from build123d import *

# Parameters (mm, degrees)
SKETCH1_R           = 1.6
BOSS_EXTRUDE1_DEPTH = 3
SKETCH2_W           = 10
SKETCH2_H           = 10
BOSS_EXTRUDE2_DEPTH = 42
CHAMFER1_SIZE       = 5
SKETCH3_R           = 2.1
CUT_EXTRUDE1_DEPTH  = 52
SKETCH4_R           = 2.65
CUT_EXTRUDE2_DEPTH  = 0.5
SKETCH5_W           = 3
SKETCH5_H           = 43
BOSS_EXTRUDE3_DEPTH = 75
SKETCH6_W           = 3
SKETCH6_H           = 72.7
BOSS_EXTRUDE4_DEPTH = 2
SKETCH7_W           = 3
SKETCH7_H           = 68.8
BOSS_EXTRUDE5_DEPTH = 3
BOSS_EXTRUDE7_DEPTH = 8.2
SKETCH9_W           = 12
SKETCH9_H           = 19.5
CUT_EXTRUDE3_DEPTH  = 8.5
SKETCH10_W          = 3
SKETCH10_H          = 56.8
BOSS_EXTRUDE8_DEPTH = 15
SKETCH13_W          = 3
SKETCH13_H          = 56.8
BOSS_EXTRUDE9_DEPTH = 45
SKETCH14_R          = 1.5
SKETCH14_R_2        = 5.5
CUT_EXTRUDE4_DEPTH  = 10
CAVITY2_START       = 23.487603306
CAVITY2_OUTLINE_R   = 2
CAVITY2_DEPTH       = 2


# Read off the part's stored shape, not the designer's step: Cavity2
with BuildPart() as part:
    # Sketch1 → Boss-Extrude1 (new body)
    with BuildSketch(Plane(origin=(0, 0, 0), x_dir=(1, 0, 0), z_dir=(0, 1, 0))):
        Polygon((-6.512396694, 9.685950413), (1.487603306, 9.685950413), (26.487603306, 9.685950413), (26.487603306, -40.314049587), (1.487603306, -40.314049587), (-6.512396694, -40.314049587), align=None)
        with Locations(Location((-1.962396694, -35.764049587, 0), (0, 0, 270))):
            Circle(SKETCH1_R, mode=Mode.SUBTRACT)
        with Locations(Location((-1.962396694, 5.135950413, 0), (0, 0, 270))):
            Circle(SKETCH1_R, mode=Mode.SUBTRACT)
    extrude(amount=BOSS_EXTRUDE1_DEPTH)

    # Sketch2 → Boss-Extrude2 (add)
    with BuildSketch(Plane(origin=(0, 3, 0), x_dir=(1, 0, 0), z_dir=(0, 1, 0))):
        with Locations((21.487603306, -35.314049587)):
            Rectangle(SKETCH2_W, SKETCH2_H)
        with Locations((21.487603306, 4.685950413)):
            Rectangle(SKETCH2_W, SKETCH2_H)
    extrude(amount=BOSS_EXTRUDE2_DEPTH)

    # Chamfer1
    chamfer1_edges = [part.edges().sort_by_distance(p)[0] for p in [
        (21.487603306, 3, 30.314049587),
        (16.487603306, 3, 35.314049587),
        (16.487603306, 3, -4.685950413),
        (21.487603306, 3, 0.314049587),
    ]]
    chamfer(chamfer1_edges, length=CHAMFER1_SIZE)

    # Sketch3 → Cut-Extrude1 (cut)
    with BuildSketch(Plane(origin=(0, 45, 0), x_dir=(1, 0, 0), z_dir=(0, 1, 0))):
        with Locations(Location((22.537603306, -36.364049587, 0), (0, 0, 270))):
            Circle(SKETCH3_R)
        with Locations(Location((22.537603306, 5.735950413, 0), (0, 0, 270))):
            Circle(SKETCH3_R)
    extrude(amount=-CUT_EXTRUDE1_DEPTH, mode=Mode.SUBTRACT)

    # Sketch4 → Cut-Extrude2 (cut)
    with BuildSketch(Plane(origin=(0, 45, 0), x_dir=(1, 0, 0), z_dir=(0, 1, 0))):
        with Locations(Location((22.537603306, -36.364049587, 0), (0, 0, 270))):
            Circle(SKETCH4_R)
        with Locations(Location((22.537603306, 5.735950413, 0), (0, 0, 270))):
            Circle(SKETCH4_R)
    cut_extrude2 = extrude(amount=-CUT_EXTRUDE2_DEPTH, mode=Mode.SUBTRACT)

    # Mirror1: Cut-Extrude2 across plane
    add(cut_extrude2.mirror(Plane(origin=(0, 22.5, 0), x_dir=(0, 0, 1), z_dir=(0, -1, 0))), mode=Mode.SUBTRACT)

    # Sketch5 → Boss-Extrude3 (add)
    with BuildSketch(Plane(origin=(0, 0, -9.685950413), x_dir=(-1, 0, 0), z_dir=(0, 0, -1))):
        with Locations((-24.987603306, 21.5)):
            Rectangle(SKETCH5_W, SKETCH5_H)
    extrude(amount=BOSS_EXTRUDE3_DEPTH)

    # Sketch6 → Boss-Extrude4 (add)
    with BuildSketch(Plane(origin=(0, 43, 0), x_dir=(1, 0, 0), z_dir=(0, 1, 0))):
        with Locations((24.987603306, 48.335950413)):
            Rectangle(SKETCH6_W, SKETCH6_H)
    extrude(amount=BOSS_EXTRUDE4_DEPTH)

    # Sketch7 → Boss-Extrude5 (add)
    with BuildSketch(Plane(origin=(0, 45, 0), x_dir=(1, 0, 0), z_dir=(0, 1, 0))):
        with Locations((24.987603306, 50.285950413)):
            Rectangle(SKETCH7_W, SKETCH7_H)
    extrude(amount=BOSS_EXTRUDE5_DEPTH)

    # Sketch8 → Boss-Extrude7 (add)
    with BuildSketch(Plane.ZY.offset(-23.487603306)):
        Polygon((-27.885950413, 24.5), (-27.885950413, 28.5), (-27.885950413, 42.5), (-29.885950413, 42.5), (-29.885950413, 22.5), (-27.885950413, 22.5), align=None)
        with BuildLine():
            Line((-15.885950413, 24.5), (-15.885950413, 28.5))
            Line((-15.885950413, 28.5), (-27.885950413, 28.5))
            Line((-27.885950413, 28.5), (-27.885950413, 24.5))
            Line((-27.885950413, 24.5), (-22.885950413, 24.5))
            ThreePointArc((-22.885950413, 24.5), (-21.885950413, 25.5), (-20.885950413, 24.5))
            Line((-20.885950413, 24.5), (-15.885950413, 24.5))
        make_face()
        with BuildLine():
            Line((-15.885950413, 22.5), (-15.885950413, 24.5))
            Line((-15.885950413, 24.5), (-20.885950413, 24.5))
            ThreePointArc((-20.885950413, 24.5), (-21.885950413, 23.5), (-22.885950413, 24.5))
            Line((-22.885950413, 24.5), (-27.885950413, 24.5))
            Line((-27.885950413, 24.5), (-27.885950413, 22.5))
            Line((-27.885950413, 22.5), (-15.885950413, 22.5))
        make_face()
        Polygon((-15.885950413, 42.5), (-15.885950413, 28.5), (-15.885950413, 24.5), (-15.885950413, 22.5), (-13.885950413, 22.5), (-13.885950413, 42.5), align=None)
    extrude(amount=BOSS_EXTRUDE7_DEPTH)

    # Sketch9 → Cut-Extrude3 (cut)
    with BuildSketch(Plane.ZY.offset(-23.487603306)):
        with Locations((-21.885950413, 38.25)):
            Rectangle(SKETCH9_W, SKETCH9_H)
    extrude(amount=-CUT_EXTRUDE3_DEPTH, mode=Mode.SUBTRACT)

    # Sketch10 → Boss-Extrude8 (add)
    with BuildSketch(Plane(origin=(0, 48, 0), x_dir=(1, 0, 0), z_dir=(0, 1, 0))):
        with Locations((24.987603306, 56.285950413)):
            Rectangle(SKETCH10_W, SKETCH10_H)
    extrude(amount=BOSS_EXTRUDE8_DEPTH)

    # Sketch13 → Boss-Extrude9 (add)
    with BuildSketch(Plane(origin=(0, 63, 0), x_dir=(1, 0, 0), z_dir=(0, 1, 0))):
        with Locations((24.987603306, 56.285950413)):
            Rectangle(SKETCH13_W, SKETCH13_H)
    extrude(amount=BOSS_EXTRUDE9_DEPTH)

    # Sketch14 → Cut-Extrude4 (cut)
    with BuildSketch(Plane.ZY.offset(-23.487603306)):
        with Locations(Location((-58.385950413, 64, 0), (0, 0, 270))):
            Circle(SKETCH14_R)
        with Locations(Location((-75.385950413, 64, 0), (0, 0, 270))):
            Circle(SKETCH14_R)
        with Locations(Location((-66.885950413, 43, 0), (0, 0, 270))):
            Circle(SKETCH14_R_2)
    extrude(amount=-CUT_EXTRUDE4_DEPTH, mode=Mode.SUBTRACT)

    # Cavity2 outline → Cavity2 (cut)
    with BuildSketch(Plane.YZ.offset(CAVITY2_START)):
        with Locations((54, -66.885950413)):
            Circle(CAVITY2_OUTLINE_R)
    extrude(amount=CAVITY2_DEPTH, mode=Mode.SUBTRACT)


solid = part.part
For this review, take the finished solid that the model builds, in its own axes (mm). A direction names the side the tool comes from. Give positions to 0.01 mm unless a question says otherwise; leave off trailing zeros. Order: outer loops, then holes, each group sorted by start corner. A loop starts at its lowest first (then second) coordinate and runs counter-clockwise, first axis right, second up. Notation, with made-up numbers: M -7.5,74.25 L 50.5,74.25 A30 cw 50.5,112.25 Z; hole C 63.5,-25 d8. An arc over 180 degrees is marked long. Answer in a Markdown table with one row per item. Add a question column.
(1) Wall thickness on probe 1 along Z at (x, y) = (18.25, 24.5); probe 2 along Z at (x, y) = (25, 64); probe 3 along Z at (x, y) = (18, 24): over which ranges is each line inside the solid? List them lowest first. Write a range as [from, to].
(2) Consider section B-B on y = 64. State the section outline as (x, z) points, and give its area (3 significant figures).
(3) Consider section C-C on y = 10.5. State the section outline as (x, z) points, and give its area (3 significant figures).
(4) For pin 1 (13 mm diameter, centred on y = 31.5, z = -19.5, fed in from -X); pin 2 (6.5 mm diameter, centred on x = 22.54, z = 36.36, fed in from +Y); pin 3 (3 mm diameter, centred on y = 17.5, z = -3, fed in from -X), all flat-tipped, find the tip position at first contact; note any pin that passes through.
(5) Consider section D-D on z = 9.5. State the section outline as (x, y) points, and give its area (3 significant figures).
(6) Mouldability with a two-part tool opening along Z and no side actions: class faces 6 (the face through (15.288, 28, -22)), 7 (the face through (-2.58, 1.48, -3.66)), 8 (the face through (25, 53, -84.686)) as +Z half, -Z half, draft (parallel to the pull), parting line (faces both ways), or undercut.
(7) For faces 1 (the face through (25.488, 54, -67)), 2 (the face through (20, 45, -4)), 3 (the face through (16.488, 26, -5)), 4 (the face through (25, 50, -27.886)), 5 (the face through (21, 44.5, -4)), list the 3-axis set-ups (+Z, -Z, +X, -X, +Y, -Y) from which the entire face can be reached by the end or side of a thin tool; tool diameter is ignored.
(8) Consider section A-A on x = 18. State the section outline as (y, z) points, and give its area (3 significant figures).
Evaluation:
| question | item | result |
|---|---|---|
| 1 | probe 1 | z = [-29.89, -22.89], [-20.89, -13.89], [-9.69, 0.31], [30.31, 40.31] |
| 1 | probe 2 | z = [-84.69, -76.89], [-73.89, -59.89], [-56.89, -27.89] |
| 1 | probe 3 | z = [-29.89, -22.75], [-21.02, -13.89], [-9.69, 0.31], [30.31, 40.31] |
| 2 | outline | M 23.49,-84.69 L 26.49,-84.69 L 26.49,-76.89 L 23.49,-76.89 Z; M 23.49,-73.89 L 26.49,-73.89 L 26.49,-59.89 L 23.49,-59.89 Z; M 23.49,-56.89 L 26.49,-56.89 L 26.49,-27.89 L 23.49,-27.89 Z |
| 2 | area | 152 mm^2 |
| 3 | outline | M 16.49,-9.69 L 23.49,-9.69 L 23.49,-84.69 L 26.49,-84.69 L 26.49,0.31 L 16.49,0.31 Z; M 16.49,30.31 L 26.49,30.31 L 26.49,40.31 L 16.49,40.31 Z; hole C 22.54,-5.74 d4.2; hole C 22.54,36.36 d4.2 |
| 3 | area | 397 mm^2 |
| 4 | pin 1 | stops at x = 15.29 |
| 4 | pin 2 | stops at y = 45 |
| 4 | pin 3 | stops at x = 16.49 |
| 5 | outline | M -6.51,0 L 26.49,0 L 26.49,3 L -6.51,3 Z |
| 5 | area | 99.0 mm^2 |
| 6 | face 6 | draft |
| 6 | face 7 | undercut |
| 6 | face 8 | -Z half |
| 7 | face 1 | -X |
| 7 | face 2 | +Z, +X, -X, +Y |
| 7 | face 3 | +Z, -X, +Y |
| 7 | face 4 | +X, -X, +Y |
| 7 | face 5 | +Y |
| 8 | outline | M 0,-9.69 L 45,-9.69 L 45,0.31 L 8,0.31 L 3,5.31 L 3,25.31 L 8,30.31 L 45,30.31 L 45,40.31 L 0,40.31 Z; M 22.5,-29.89 L 42.5,-29.89 L 42.5,-27.89 L 28.5,-27.89 L 28.5,-15.89 L 42.5,-15.89 L 42.5,-13.89 L 22.5,-13.89 Z; hole C 24.5,-21.89 d2 |
| 8 | area | 1,160 mm^2 |
